Build history of the part. All positions in model axes, mm. Round coordinates to 2 decimals unless told otherwise and drop trailing zeros. Order: outer loops, then holes, each group sorted by start corner. A loop starts at its lowest first (then second) coordinate and runs counter-clockwise, first axis right, second up. Notation, with made-up numbers: M 21,70.5 L 64,70.5 A29 ccw 64,100.5 Z; hole C 39.5,40.25 d4. An arc over 180 degrees is marked long. Use CSV: the item, a comma, the result in double quotes.
from build123d import *

# Parameters (mm, degrees)
F0_R     = 6
F0_R_2   = 30
F0_R_3   = 3.5
F1_DEPTH = 2.5


# Not quite as in the source:
# - a feature names something its author has since deleted; it is built from what else it names


with BuildPart() as f1:
    # F0 (on Front) → F1 (new body, symmetric)
    with BuildSketch(Plane.XZ):
        Polygon((0, 255), (1435, 0), (1435, 547.5993031359), (-565, 903), (-565, 355.4006968641), align=None)
        with Locations((335.4070785648, 292.4334004787)):
            Circle(F0_R, mode=Mode.SUBTRACT)
        with Locations((335.4070785648, 407.4334004787)):
            Circle(F0_R, mode=Mode.SUBTRACT)
        with Locations((435, 234.9334004787)):
            Circle(F0_R, mode=Mode.SUBTRACT)
        with Locations((534.5929214352, 292.4334004787)):
            Circle(F0_R, mode=Mode.SUBTRACT)
        with Locations((435, 349.9334004787)):
            Circle(F0_R_2, mode=Mode.SUBTRACT)
        with Locations((534.5929214352, 407.4334004787)):
            Circle(F0_R, mode=Mode.SUBTRACT)
        with Locations((857.3829507159, 447.1088550113)):
            Circle(F0_R_3, mode=Mode.SUBTRACT)
        with Locations((998.1772676211, 422.08965584)):
            Circle(F0_R_3, mode=Mode.SUBTRACT)
        with Locations((1138.9715845264, 397.0704566686)):
            Circle(F0_R_3, mode=Mode.SUBTRACT)
        with Locations((1279.7659014317, 372.0512574973)):
            Circle(F0_R_3, mode=Mode.SUBTRACT)
        with Locations((1420.560218337, 347.032058326)):
            Circle(F0_R_3, mode=Mode.SUBTRACT)
        with Locations((1420.560218337, 448.5986578473)):
            Circle(F0_R_3, mode=Mode.SUBTRACT)
        with Locations((-409.7659014317, 672.2816475532)):
            Circle(F0_R_3, mode=Mode.SUBTRACT)
        with Locations((-268.9715845264, 647.2624483819)):
            Circle(F0_R_3, mode=Mode.SUBTRACT)
        with Locations((-128.1772676211, 622.2432492105)):
            Circle(F0_R_3, mode=Mode.SUBTRACT)
        with Locations((294.2056830947, 547.1856516966)):
            Circle(F0_R_3, mode=Mode.SUBTRACT)
        with Locations((12.6170492841, 597.2240500392)):
            Circle(F0_R_3, mode=Mode.SUBTRACT)
        with Locations((153.4113661894, 572.2048508679)):
            Circle(F0_R_3, mode=Mode.SUBTRACT)
        with Locations((153.4113661894, 673.7714503892)):
            Circle(F0_R_3, mode=Mode.SUBTRACT)
        with Locations((294.2056830947, 648.7522512179)):
            Circle(F0_R_3, mode=Mode.SUBTRACT)
        with Locations((-550.560218337, 697.3008467245)):
            Circle(F0_R_3, mode=Mode.SUBTRACT)
        with Locations((-409.7659014317, 773.8482470745)):
            Circle(F0_R_3, mode=Mode.SUBTRACT)
        with Locations((-128.1772676211, 723.8098487319)):
            Circle(F0_R_3, mode=Mode.SUBTRACT)
        with Locations((-268.9715845264, 748.8290479032)):
            Circle(F0_R_3, mode=Mode.SUBTRACT)
        with Locations((-550.560218337, 798.8674462459)):
            Circle(F0_R_3, mode=Mode.SUBTRACT)
        with Locations((12.6170492841, 698.7906495606)):
            Circle(F0_R_3, mode=Mode.SUBTRACT)
        with Locations((435, 464.9334004787)):
            Circle(F0_R, mode=Mode.SUBTRACT)
        with Locations((575.7943169053, 497.1472533539)):
            Circle(F0_R_3, mode=Mode.SUBTRACT)
        with Locations((435, 522.1664525253)):
            Circle(F0_R_3, mode=Mode.SUBTRACT)
        with Locations((716.5886338106, 472.1280541826)):
            Circle(F0_R_3, mode=Mode.SUBTRACT)
        with Locations((857.3829507159, 548.6754545326)):
            Circle(F0_R_3, mode=Mode.SUBTRACT)
        with Locations((575.7943169053, 598.7138528753)):
            Circle(F0_R_3, mode=Mode.SUBTRACT)
        with Locations((435, 623.7330520466)):
            Circle(F0_R_3, mode=Mode.SUBTRACT)
        with Locations((716.5886338106, 573.694653704)):
            Circle(F0_R_3, mode=Mode.SUBTRACT)
        with Locations((1138.9715845264, 498.63705619)):
            Circle(F0_R_3, mode=Mode.SUBTRACT)
        with Locations((998.1772676211, 523.6562553613)):
            Circle(F0_R_3, mode=Mode.SUBTRACT)
        with Locations((1279.7659014317, 473.6178570187)):
            Circle(F0_R_3, mode=Mode.SUBTRACT)
    extrude(amount=F1_DEPTH, both=True)


solid = f1.part
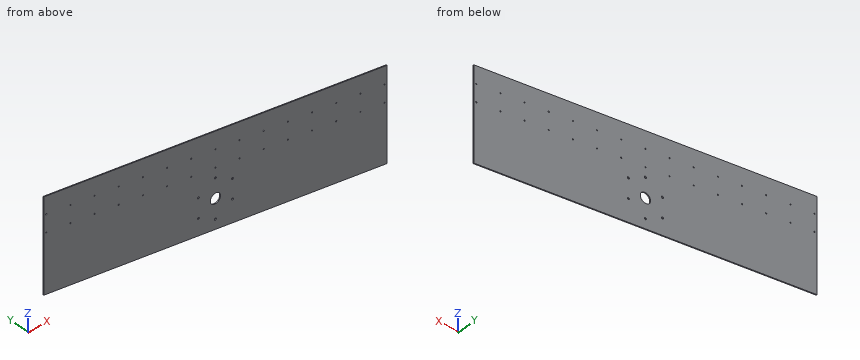
(1) Drop a flat-ended pin along its axis: pin 1 (6.5 mm diameter, centred on x = 1279.77, z = 372.05, fed in from +Y). Give the stop position or say it passes through.
Answer block:
pin 1,"passes through"
(2) Cut at A-A, the plane x = 964.5. Give the cut face in (y, z), and give its area (3 significant figures).
Answer block:
outline,"M -2.5,83.61 L 2.5,83.61 L 2.5,631.21 L -2.5,631.21 Z"
area,"2,740 mm²"
(3) Cut at B-B, the plane y = -1.1. Count the separate pieces of the cut face and the enclosed holes in it, and give its area (3 significant figures).
Answer block:
separate pieces,"1"
enclosed holes,"37"
area,"1,090,000 mm²"
(4) Wall check: line 1 (Z direction, x = 435, y = -1.1); line 2 (Z direction, x = -446.5, y = -0.45); line 3 (Z direction, x = 774, y = -0.5). Give the ranges that are in metal, low to high. Write a range as from..to.
Answer block:
line 1,"z = 177.7..228.93, 240.93..319.93, 379.93..458.93, 470.93..518.67, 525.67..620.23, 627.23..725.3"
line 2,"z = 334.34..881.94"
line 3,"z = 117.46..665.06"
